from build123d import *

# Parameters (mm, degrees)
F0_W     = 30.48
F0_H     = 25.4
F0_W_2   = 25.4
F0_H_2   = 20.32
F1_DEPTH = 31.75
F2_W     = 25.4
F2_H     = 20.32
F2_W_2   = 20.32
F2_H_2   = 15.24
F2_R     = 2.159
F3_DEPTH = 12.7
F4_R     = 2.159
F5_DEPTH = 5.08


with BuildPart() as f1:
    # F0 (on Top) → F1 (new body, symmetric)
    with BuildSketch(Plane.XY):
        Rectangle(F0_W, F0_H)
        Rectangle(F0_W_2, F0_H_2, mode=Mode.SUBTRACT)
    extrude(amount=F1_DEPTH, both=True)

    # F2 (on face) → F3 (join)
    with BuildSketch(Plane.XY.offset(31.75)):
        Rectangle(F2_W, F2_H)
        Rectangle(F2_W_2, F2_H_2, mode=Mode.SUBTRACT)
        Rectangle(F2_W_2, F2_H_2)
        with Locations((-6.35, 0)):
            Circle(F2_R, mode=Mode.SUBTRACT)
        with Locations((6.35, 0)):
            Circle(F2_R, mode=Mode.SUBTRACT)
    extrude(amount=-F3_DEPTH)

    # F4 (on face) → F5 (cut)
    with BuildSketch(Plane(origin=(0, 0, 19.05), x_dir=(1, 0, 0), z_dir=(0, 0, -1))):
        Polygon((-3.683, 4.6193795038), (-9.017, 4.6193795038), (-11.684, 0), (-9.017, -4.6193795038), (-3.683, -4.6193795038), (-1.016, 0), align=None)
        with Locations((-6.35, 0)):
            Circle(F4_R, mode=Mode.SUBTRACT)
        Polygon((9.017, 4.6193795038), (3.683, 4.6193795038), (1.016, 0), (3.683, -4.6193795038), (9.017, -4.6193795038), (11.684, 0), align=None)
        with Locations((6.35, 0)):
            Circle(F4_R, mode=Mode.SUBTRACT)
        with Locations((-6.35, 0)):
            Circle(F4_R)
        with Locations((6.35, 0)):
            Circle(F4_R)
    extrude(amount=-F5_DEPTH, mode=Mode.SUBTRACT)


solid = f1.part
Design review of the part built by this model. Coordinates are the model's own, in mm. A direction names the side the tool comes from. Give positions to 0.01 mm unless a question says otherwise; leave off trailing zeros. Write each loop counter-clockwise with the first axis right and the second up, starting at its lowest first coordinate (ties: lowest second). Pieces come first, ordered by that corner, then holes. Notation, with made-up numbers: M 44,26 L 92,26 A25 cw 92,42 Z; hole C 75.25,-29 d3. An arc over 180 degrees is marked long. Return JSON: item names as keys, results as strings. Group by question number.
Item 1: Take a section at A-A (z = 8). Give the boundary of the cut face in (x, y).
Item 2: Clearance check with flat-ended pins moving along their axes: pin 1 Ø3 at (x, y) = (-10.5, -1.5) entering from -Z; pin 2 Ø4.5 at (x, y) = (-8.5, -0.5) entering from -Z. State where each tip first meets the part, or that it passes through.
Item 3: Take a section at B-B (y = -9.5). Give the boundary of the cut face in (x, z).
Item 4: Take a section at D-D (x = -10.5). Give the boundary of the cut face in (y, z), plus the area to 3 significant figures.
Item 5: Take a section at C-C (x = 6.35). Give the boundary of the cut face in (y, z).
Item 6: The part is to be moulded in two halves that separate along Y. For faces 1 (the flat face through (0, 12.7, 0)), 2 (the flat face through (-15.24, 0, 0)), 3 (the flat face through (0, -12.7, 0)), 4 (the flat face through (-2.368, 2.342, 21.554)), say which applies: pulls with the +Y half, pulls with the -Y half, needs draft (parallel to the pull), parting line crosses it, or undercut.
Item 7: Wall thickness on line 1 along X through (y, z) = (8, 12); line 2 along Y through (x, z) = (-4.5, 1); line 3 along Z through (x, y) = (8.5, 3.75): over which ranges is each line inside the solid? List them lowest first.
Item 8: Tool access review of faces 5 (the flat face through (-4, 0, 24.13)), 6 (the flat face through (15.24, 0, 0)): name each direction out of +Z, -Z, +X, -X, +Y, -Y from which nothing blocks a thin tool from reaching the whole face with its end or side.
Return value:
{
 "1": {"outline": "M -15.24,-12.7 L 15.24,-12.7 L 15.24,12.7 L -15.24,12.7 Z; hole M -12.7,-10.16 L 12.7,-10.16 L 12.7,10.16 L -12.7,10.16 Z"},
 "2": {"pin 1": "stops at z = 19.05", "pin 2": "stops at z = 24.13"},
 "3": {"outline": "M -15.24,-31.75 L -12.7,-31.75 L -12.7,19.05 L 12.7,19.05 L 12.7,-31.75 L 15.24,-31.75 L 15.24,31.75 L -15.24,31.75 Z"},
 "4": {"outline": "M -12.7,-31.75 L -10.16,-31.75 L -10.16,19.05 L -2.05,19.05 L -2.05,24.13 L 2.05,24.13 L 2.05,19.05 L 10.16,19.05 L 10.16,-31.75 L 12.7,-31.75 L 12.7,31.75 L -12.7,31.75 Z", "area": "560 mm2"},
 "5": {"outline": "M -12.7,-31.75 L -10.16,-31.75 L -10.16,19.05 L -4.62,19.05 L -4.62,24.13 L -2.16,24.13 L -2.16,31.75 L -12.7,31.75 Z; M 2.16,24.13 L 4.62,24.13 L 4.62,19.05 L 10.16,19.05 L 10.16,-31.75 L 12.7,-31.75 L 12.7,31.75 L 2.16,31.75 Z"},
 "6": {"face 1": "pulls with the +Y half", "face 2": "needs draft", "face 3": "pulls with the -Y half", "face 4": "undercut"},
 "7": {"line 1": "x = -15.24 to -12.7, 12.7 to 15.24", "line 2": "y = -12.7 to -10.16, 10.16 to 12.7", "line 3": "z = 24.13 to 31.75"},
 "8": {"face 5": "-Z", "face 6": "+Z, -Z, +X, +Y, -Y"}
}
